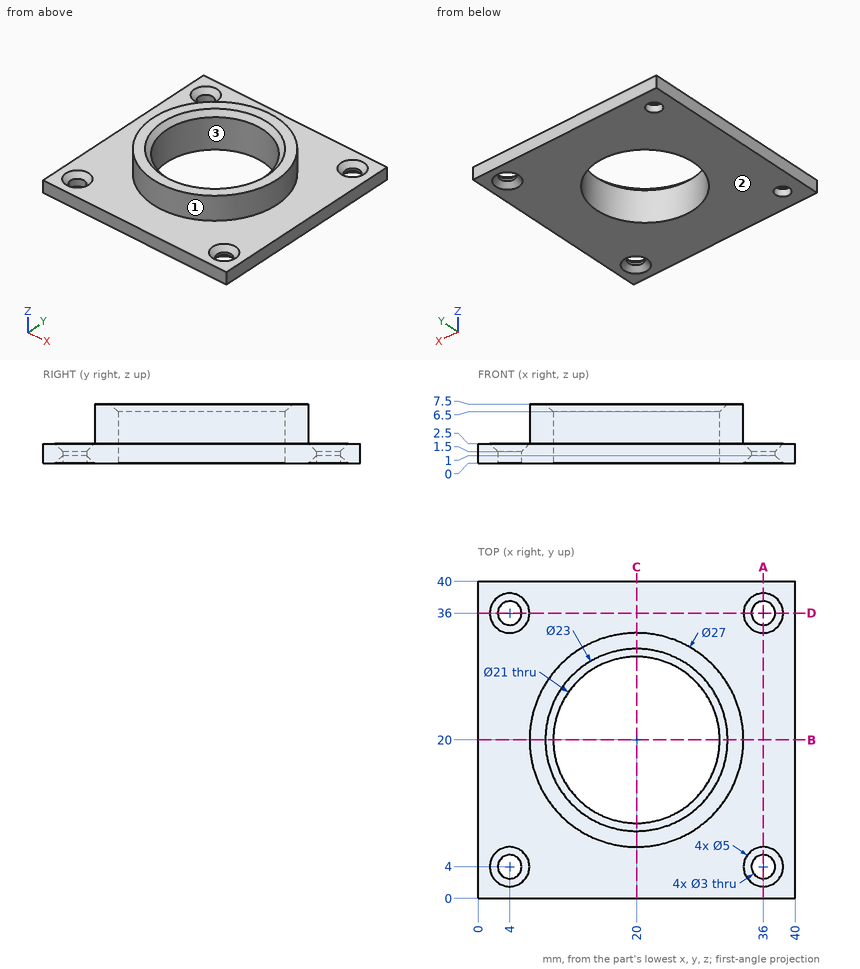
Part print with two shaded views. Sizes in mm from the minimum x, y, z corner. Round coordinates to 2 decimals unless told otherwise and drop trailing zeros. Write each loop counter-clockwise with the first axis right and the second up, starting at its lowest first coordinate (ties: lowest second). Pieces come first, ordered by that corner, then holes. Notation, with made-up numbers: M 58.25,-5 L 87.25,-5 A18 cw 87.25,23 Z; hole C 35.25,13 d5. An arc over 180 degrees is marked long. Use CSV: the item, a comma, the result in double quotes.
1. Wall check: probe 1 along Y at (x, z) = (36, 1.1); probe 2 along Z at (x, y) = (11, 34); probe 3 along X at (y, z) = (16.5, 7). Give the ranges that are in metal, low to high. Write a range as from..to.
Reply:
probe 1,"y = 0..2.5, 5.5..34.5, 37.5..40"
probe 2,"z = 0..2.5"
probe 3,"x = 6.96..9.57, 30.43..33.04"
2. Flat gauge pins, fed straight in: pin 1 (3 mm diameter, centred on x = 9, z = 5, fed in from +Y); pin 2 (4 mm diameter, centred on y = 26, z = 5, fed in from +X); pin 3 (2 mm diameter, centred on y = 26.5, z = 6, fed in from -X). Where does each tip first touch, or does it go through?
Reply:
pin 1,"stops at y = 29.59"
pin 2,"stops at x = 32.89"
pin 3,"stops at x = 7.67"
3. Saw through at A-A (x = 36). Give the cut face in (y, z).
Reply:
outline,"M 0,0 L 1.5,0 L 2.5,1 L 2.5,1.5 L 1.5,2.5 L 0,2.5 Z; M 5.5,1 L 6.5,0 L 33.5,0 L 34.5,1 L 34.5,1.5 L 33.5,2.5 L 6.5,2.5 L 5.5,1.5 Z; M 37.5,1 L 38.5,0 L 40,0 L 40,2.5 L 38.5,2.5 L 37.5,1.5 Z"
4. Saw through at D-D (y = 36). Give the cut face in (x, z).
Reply:
outline,"M 0,0 L 2.5,0 L 2.5,1.5 L 1.5,2.5 L 0,2.5 Z; M 5.5,0 L 33.5,0 L 34.5,1 L 34.5,1.5 L 33.5,2.5 L 6.5,2.5 L 5.5,1.5 Z; M 37.5,1 L 38.5,0 L 40,0 L 40,2.5 L 38.5,2.5 L 37.5,1.5 Z"
5. Saw through at B-B (y = 20). Give the cut face in (x, z).
Reply:
outline,"M 0,0 L 9.5,0 L 9.5,6.5 L 8.5,7.5 L 6.5,7.5 L 6.5,2.5 L 0,2.5 Z; M 30.5,0 L 40,0 L 40,2.5 L 33.5,2.5 L 33.5,7.5 L 31.5,7.5 L 30.5,6.5 Z"
6. Two-plate mould, pull along Y, no slides. Class the marked faces 1, 2 and 3: +Y half, -Y half, draft (parallel to the pull), parting line (faces both ways), or undercut.
Reply:
face 1,"parting line"
face 2,"draft"
face 3,"undercut"
